from build123d import *

# Parameters (mm, degrees)
F0_R            = 50
F1_DEPTH        = 20
F2_R            = 13
F3_DEPTH        = 20
F5_DEPTH        = 19.5
F5_COPIES_COUNT = 12


# Not quite as in the source:
# - a pattern or mirror of a feature is missing from the dataset's text; its kind, count and spacing are read off the source's solid


with BuildPart() as f1:
    # F0 (on Top) → F1 (new body)
    with BuildSketch(Plane.XY):
        Circle(F0_R)
    extrude(amount=F1_DEPTH)

    # F2 (on Top) → F3 (cut)
    with BuildSketch(Plane.XY):
        Circle(F2_R)
    extrude(amount=F3_DEPTH, mode=Mode.SUBTRACT)

    # F4 (on Top) → F5 (join)
    with BuildSketch(Plane.XY):
        with BuildLine():
            Line((0, 70.5249483342), (-11.9310349513, 48.55564236))
            ThreePointArc((-11.9310349513, 48.55564236), (0, 50), (11.9310349513, 48.55564236))
            Line((11.9310349513, 48.55564236), (0, 70.5249483342))
        make_face()
    f5 = extrude(amount=F5_DEPTH)

    # F5_copies: F5 ×12 about axis
    f5_copies_axis = Axis((0, 0, 0), (0, 0, 1))
    for i in range(1, F5_COPIES_COUNT):
        add(f5.rotate(f5_copies_axis, i * 360 / F5_COPIES_COUNT))


solid = f1.part
Input: part model. Units: mm. Frame: model coordinates. A direction names the side the tool comes from. Give positions to 0.01 mm unless a question says otherwise; leave off trailing zeros. Order: outer loops, then holes, each group sorted by start corner. A loop starts at its lowest first (then second) coordinate and runs counter-clockwise, first axis right, second up. Notation, with made-up numbers: (87.5, 7.5) - (139.5, 7.5) arc R12 cw to (139.5, 26.5) - close; hole circle Ø8 at (61.25, -33). An arc over 180 degrees is marked (long way). Write each question's results on one line, items separated by ' | '.
Item 1: Section A-A (x = 56.5). Return loops of the section in (y, z).
A:
outline: (-35.14, 0) - (-27.79, 0) - (-27.79, 19.5) - (-35.14, 19.5) - close; (-7.62, 0) - (7.62, 0) - (7.62, 19.5) - (-7.62, 19.5) - close; (27.79, 0) - (35.14, 0) - (35.14, 19.5) - (27.79, 19.5) - close
Item 2: Access query for faces 1 (the flat face through (-50, 28, 19.5)), 2 (the flat face through (-59.694, -5.882, 9.614)), 3 (the flat face through (-28, -50, 19.5)). Directions: +Z, -Z, +X, -X, +Y, -Y. A direction counts if a zero-diameter tool reaches every point of the face in a straight line with its end or side. Return the directions, or none.
A:
face 1: +Z, -X, +Y | face 2: +Z, -Z, -X | face 3: +Z, -X, -Y
Item 3: Contact query for flat-ended pins moving along their axis: pin 1 Ø21 at (x, y) = (0, 0) entering from +Z; pin 2 Ø10.5 at (x, y) = (24, -51) entering from +Z; pin 3 Ø5 at (x, z) = (50, 10) entering from -Y; pin 4 Ø5 at (y, z) = (-40, 17.5) entering from +X. Output: stop coordinate, or through.
A:
pin 1: passes through | pin 2: stops at z = 19.5 | pin 3: stops at y = -35.04 | pin 4: stops at x = 34.78
Item 4: Section C-C (y = 33). Return loops of the section in (x, z).
A:
outline: (-59.69, 0) - (59.69, 0) - (59.69, 19.5) - (37.56, 19.5) - (37.56, 20) - (-37.56, 20) - (-37.56, 19.5) - (-59.69, 19.5) - close
Item 5: Section D-D (x = -26). Return loops of the section in (y, z), and give its area (3 significant figures).
A:
outline: (-55.4, 0) - (55.4, 0) - (55.4, 19.5) - (42.71, 19.5) - (42.71, 20) - (-42.71, 20) - (-42.71, 19.5) - (-55.4, 19.5) - close | area: 2,200 mm^2
Item 6: Section B-B (y = 57). Return loops of the section in (x, z), and give its area (3 significant figures).
A:
outline: (-35.16, 0) - (-28.61, 0) - (-28.61, 19.5) - (-35.16, 19.5) - close; (-7.35, 0) - (7.35, 0) - (7.35, 19.5) - (-7.35, 19.5) - close; (28.61, 0) - (35.16, 0) - (35.16, 19.5) - (28.61, 19.5) - close | area: 542 mm^2
Item 7: Material intervals for line 1 along Y through (x, z) = (0, 14.25); line 2 along Y through (x, z) = (-54, 2); line 3 along Y through (x, z) = (52, 16.5), sorted ascending.
A:
line 1: y = -70.52 to -13, 13 to 70.52 | line 2: y = -35.08 to -23.71, -8.97 to 8.97, 23.71 to 35.08 | line 3: y = -35.03 to -20.45, -10.06 to 10.06, 20.45 to 35.03
Item 8: Draft query along Y for faces 4 (the flat face through (59.694, 5.882, 9.614)), 5 (the flat face through (28, 50, 19.5)), 6 (the flat face through (-5.882, 59.694, 9.614)). Return one class per face: released by +Y, released by -Y, zero draft, split by the parting line, or undercut.
A:
face 4: undercut | face 5: zero draft | face 6: released by +Y
